```python
from build123d import *

# Parameters (mm, degrees)
F0_R     = 1.6
F1_DEPTH = 3
F2_W     = 3.05
F2_H     = 6
F3_DEPTH = 3
F5_D     = 1
F6_R     = 1


with BuildPart() as f1:
    # F0 (on Top) → F1 (new body)
    with BuildSketch(Plane.XY):
        with BuildLine():
            Line((-20, 0), (-20, -7.5))
            Line((-20, -7.5), (-13.9, -7.5))
            Line((-13.9, -7.5), (-13.9, -10.6))
            Line((-13.9, -10.6), (13.9, -10.6))
            Line((13.9, -10.6), (13.9, -7.5))
            Line((13.9, -7.5), (20, -7.5))
            Line((20, -7.5), (20, 0))
            Line((20, 0), (20, 7.5))
            Line((20, 7.5), (17, 7.5))
            ThreePointArc((17, 7.5), (15.615651922, 8.0992038794), (15.1050482082, 9.5186223298))
            ThreePointArc((15.1050482082, 9.5186223298), (5.125, 20.15), (-4.8550482082, 9.5186223298))
            ThreePointArc((-4.8550482082, 9.5186223298), (-5.365651922, 8.0992038794), (-6.75, 7.5))
            Line((-6.75, 7.5), (-20, 7.5))
            Line((-20, 7.5), (-20, 0))
        make_face()
        with Locations((-15, 0)):
            Circle(F0_R, mode=Mode.SUBTRACT)
        with Locations((15, 0)):
            Circle(F0_R, mode=Mode.SUBTRACT)
        with BuildLine():
            ThreePointArc((-0.325, 9.6), (-0.875, 10.15), (-0.325, 10.7))
            Line((-0.325, 10.7), (10.575, 10.7))
            ThreePointArc((10.575, 10.7), (10.9639087297, 10.5389087297), (11.125, 10.15))
            ThreePointArc((11.125, 10.15), (10.9639087297, 9.7610912703), (10.575, 9.6))
            Line((10.575, 9.6), (-0.325, 9.6))
        make_face(mode=Mode.SUBTRACT)
    extrude(amount=F1_DEPTH)

    # F2 (on face) → F3 (join, through all)
    with BuildSketch(Plane.XY.offset(3)):
        with Locations((-21.525, 0)):
            Rectangle(F2_W, F2_H)
        with Locations((21.525, 0)):
            Rectangle(F2_W, F2_H)
    extrude(amount=-F3_DEPTH)

    # F5 (through all)
    with Locations(Plane.XY.offset(3)):
        with Locations((13.9, -7.5), (20, -3), (20, 3), (-13.9, -7.5), (-20, -3), (-20, 3)):
            Hole(F5_D / 2)

    # F6
    f6_edges = [f1.edges().sort_by_distance(p)[0] for p in [
        (20, 7.5, 1.5),
        (23.05, 3, 1.5),
        (23.05, -3, 1.5),
        (13.9, -10.6, 1.5),
        (20, -7.5, 1.5),
        (-23.05, 3, 1.5),
        (-20, 7.5, 1.5),
        (-20, -7.5, 1.5),
        (-13.9, -10.6, 1.5),
        (-23.05, -3, 1.5),
        (20, 3.5, 1.5),
        (20.5, 3, 1.5),
        (20.5, -3, 1.5),
        (20, -3.5, 1.5),
        (14.4, -7.5, 1.5),
        (13.9, -8, 1.5),
        (-13.9, -8, 1.5),
        (-14.4, -7.5, 1.5),
        (-20, -3.5, 1.5),
        (-20.5, -3, 1.5),
        (-20.5, 3, 1.5),
        (-20, 3.5, 1.5),
    ]]
    fillet(f6_edges, radius=F6_R)


solid = f1.part
```
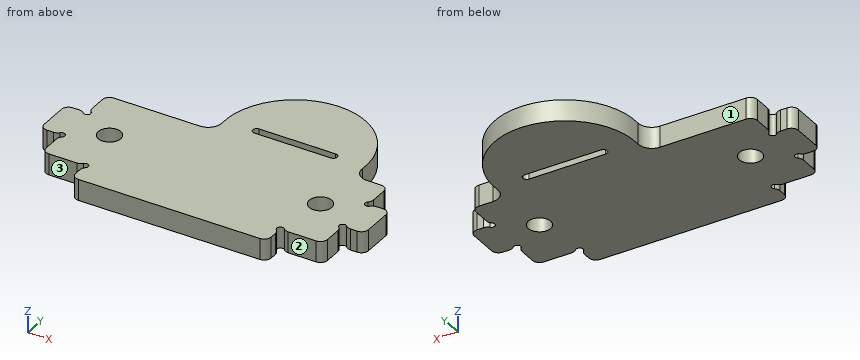
The listing builds one solid part. Answer for the finished solid, in the listing's coordinates (mm). Face numbers are marked on the shaded views. A direction names the side the tool comes from. Round coordinates to 2 decimals unless told otherwise and drop trailing zeros. Loops run counter-clockwise (first coordinate to the right, second up) from the corner with the lowest first, then second, coordinate; pieces in that order, holes last.
1) A cutting plane is placed at A-A on y = 0. Determine the outline of the cut face in (x, z).
Outcome:
outline: (-23.05, 0) - (-16.6, 0) - (-16.6, 3) - (-23.05, 3) - close; (-13.4, 0) - (13.4, 0) - (13.4, 3) - (-13.4, 3) - close; (16.6, 0) - (23.05, 0) - (23.05, 3) - (16.6, 3) - close
2) A cutting plane is placed at C-C on z = 2.55. Give the number of separate pieces and of enclosed holes in the cut face, plus the area to 3 significant figures.
Outcome:
separate pieces: 1
enclosed holes: 3
area: 899 mm2
3) A cutting plane is placed at D-D on x = -18. Determine the outline of the cut face in (y, z).
Outcome:
outline: (-7.5, 0) - (7.5, 0) - (7.5, 3) - (-7.5, 3) - close
4) For the marked faces 1, 2 and 3, determine the directions among +Z, -Z, +X, -X, +Y, -Y from which every point of the face is accessible in a straight line to the end or side of a thin tool.
Outcome:
face 1: +Z, -Z, -X, +Y
face 2: +Z, -Z, +X, -Y
face 3: +Z, -Z, -X, -Y
5) Given P1, Ø1.5, axis at x = 7.5, z = 2, coming from the +Y side; P2, Ø1, axis at x = 17.5, z = 1, coming from the +Y side; P3, Ø0.7, axis at x = -21.5, z = 2, coming from the +Y side; P4, Ø3, axis at x = 15, y = 0, coming from the -Z side (3 decimals), each flat-ended and moving along its own axis, determine where each tip first touches the part or whether it passes through.
Outcome:
P1: stops at y = 20.02
P2: stops at y = 7.5
P3: stops at y = 3
P4: passes through
6) A cutting plane is placed at B-B on x = 5. Determine the outline of the cut face in (y, z).
Outcome:
outline: (-10.6, 0) - (9.6, 0) - (9.6, 3) - (-10.6, 3) - close; (10.7, 0) - (20.15, 0) - (20.15, 3) - (10.7, 3) - close
7) Consider line 1 (X direction, y = -0.5, z = 1.2); line 2 (Y direction, x = -15, z = 1.6); line 3 (Y direction, x = -7, z = 2.5). Determine where each line is inside the solid, lowest interval first.
Outcome:
line 1: x = -23.05 to -16.52, -13.48 to 13.48, 16.52 to 23.05
line 2: y = -7.5 to -1.6, 1.6 to 7.5
line 3: y = -10.6 to 7.5
